Work out the finished part from the listing and answer in its coordinate system (mm). A direction names the side the tool comes from. Give positions to 0.01 mm unless a question says otherwise; leave off trailing zeros. Write each loop counter-clockwise with the first axis right and the second up, starting at its lowest first coordinate (ties: lowest second). Pieces come first, ordered by that corner, then holes. Notation, with made-up numbers: (-28, 12) - (5, 12) arc R20 cw to (5, 45) - close; hole circle Ø6 at (55, 62). An arc over 180 degrees is marked (long way). Write item = value, one per line.
from build123d import *

# Parameters (mm, degrees)
F0_W     = 50.8
F0_H     = 50.8
F2_DEPTH = 203.2
F1_W     = 44.45
F1_H     = 44.45
F3_DEPTH = 203.2


with BuildPart() as f2:
    # F0 (on Top) → F2 (new body)
    with BuildSketch(Plane.XY):
        Rectangle(F0_W, F0_H)
    extrude(amount=F2_DEPTH)

    # F1 (on Top) → F3 (cut)
    with BuildSketch(Plane.XY):
        Rectangle(F1_W, F1_H)
    extrude(amount=F3_DEPTH, mode=Mode.SUBTRACT)


solid = f2.part
1. A straight line is drawn through the part: line 1 (X direction, y = -7.5, z = 131) (3 decimals). Find the intervals that lie inside material, in ascending order.
Solution:
line_1 = -25.4 to -22.225, 22.225 to 25.4
2. Find section A-A, the plane y = 13. Give the vertices of the cut face in (x, z) (3 decimals), then the cut area to 3 significant figures.
Solution:
outline = (-25.4, 0) - (-22.225, 0) - (-22.225, 203.2) - (-25.4, 203.2) - close; (22.225, 0) - (25.4, 0) - (25.4, 203.2) - (22.225, 203.2) - close
area = 1,290 mm^2
3. Find section C-C, the plane z = 56.5. Give the vertices of the cut face in (x, y) (3 decimals), then the cut area to 3 significant figures.
Solution:
outline = (-25.4, -25.4) - (25.4, -25.4) - (25.4, 25.4) - (-25.4, 25.4) - close; hole (-22.225, -22.225) - (22.225, -22.225) - (22.225, 22.225) - (-22.225, 22.225) - close
area = 605 mm^2
4. For a pull along X with two mould halves and no side action, classify faces 1 (the flat face through (25.4, 0, 100)), 2 (the flat face through (-23, 0, 203.2)), 3 (the flat face through (22.225, 0, 100)), 4 (the flat face through (0, -22.225, 100)) as pulls with the +X half, pulls with the -X half, needs draft (parallel to the pull), parting line crosses it, or undercut.
Solution:
face_1 = pulls with the +X half
face_2 = needs draft
face_3 = undercut
face_4 = undercut
5. A tool of negligible diameter and unlimited length cuts with its end or side. For faces 5 (the flat face through (-22.225, 0, 100)), 6 (the flat face through (-23, 0, 0)), from which of +Z, -Z, +X, -X, +Y, -Y can it reach the whole face along a straight path? Write none if from no direction.
Solution:
face_5 = +Z, -Z
face_6 = -Z, +X, -X, +Y, -Y
